from build123d import *

# Parameters (mm, degrees)
EXTRUDE_1_DEPTH     = 40
CUT_EXTRUDE_1_REACH = 130.577
CUT_EXTRUDE_2_REACH = 130.577


with BuildPart() as part:
    # 草图1 → 凸台-拉伸1 (new body)
    with BuildSketch(Plane(origin=(0, 0, 0), x_dir=(0, 0, -1), z_dir=(1, 0, 0))):
        Polygon((0, 0), (0, 114), (44, 114), (44, 110), (4, 110), (4, 0), align=None)
    extrude(amount=EXTRUDE_1_DEPTH)

    # 草图2 → 切除-拉伸1 (cut, up to next)
    with BuildSketch(Plane(origin=(0, 114, 0), x_dir=(1, 0, 0), z_dir=(0, 1, 0)), mode=Mode.PRIVATE) as cut_extrude_1_sk1:
        with BuildLine():
            Line((17, 32), (17, 17))
            ThreePointArc((17, 17), (20, 14), (23, 17))
            Line((23, 17), (23, 32))
            ThreePointArc((23, 32), (20, 35), (17, 32))
        make_face()
    cut_extrude_1_tool1 = extrude(cut_extrude_1_sk1.sketch, amount=-CUT_EXTRUDE_1_REACH, mode=Mode.PRIVATE) & part.part
    add(cut_extrude_1_tool1.solids().sort_by_distance((20, 114, -24.5))[0], mode=Mode.SUBTRACT)

    # 草图3 → 切除-拉伸2 (cut, up to next)
    with BuildSketch(Plane.XY, mode=Mode.PRIVATE) as cut_extrude_2_sk1:
        with BuildLine():
            Line((23.5, 15), (23.5, 35))
            ThreePointArc((23.5, 35), (20, 38.5), (16.5, 35))
            Line((16.5, 35), (16.5, 15))
            ThreePointArc((16.5, 15), (20, 11.5), (23.5, 15))
        make_face()
    cut_extrude_2_tool1 = extrude(cut_extrude_2_sk1.sketch, amount=-CUT_EXTRUDE_2_REACH, mode=Mode.PRIVATE) & part.part
    add(cut_extrude_2_tool1.solids().sort_by_distance((20, 25, 0))[0], mode=Mode.SUBTRACT)


solid = part.part
Here's how the part is built. I have some questions about the finished solid (model axes, mm). A direction names the side the tool comes from. Coordinates: 2 decimals unless noted, no trailing zeros. Write each loop counter-clockwise with the first axis right and the second up, starting at its lowest first coordinate (ties: lowest second). Pieces come first, ordered by that corner, then holes. Notation, with made-up numbers: (47.5, -40) - (58.5, -40) arc R18 ccw to (58.5, -11) - close; hole circle Ø5 at (76, 17). An arc over 180 degrees is marked (long way). Use one line per item in the form item = value.
1) Suppose I cut it at D-D, the plane y = 47. Write out the boundary of the cut face in (x, z), plus the area to 3 significant figures.
Solved:
outline = (0, -4) - (40, -4) - (40, 0) - (0, 0) - close
area = 160 mm2
2) I need wall thicknesses on line 1 (Y direction, x = 22, z = -41); line 2 (Z direction, x = 31, y = 83). Which ranges of each line are inside material? Lowest first, please.
Solved:
line_1 = 110 to 114
line_2 = -4 to 0
3) Suppose I cut it at B-B, the plane y = 19. Write out the boundary of the cut face in (x, z).
Solved:
outline = (0, -4) - (16.5, -4) - (16.5, 0) - (0, 0) - close; (23.5, -4) - (40, -4) - (40, 0) - (23.5, 0) - close
4) I'm going to push flat-ended pins straight in: P1, Ø4, axis at x = 11, z = -30.5, coming from the -Y side; P2, Ø12, axis at x = 24, y = 46.5, coming from the -Z side. Where does each tip first touch, or does it pass through?
Solved:
P1 = 110
P2 = -4
5) Suppose I cut it at C-C, the plane x = 20. Write out the boundary of the cut face in (y, z).
Solved:
outline = (0, -4) - (11.5, -4) - (11.5, 0) - (0, 0) - close; (38.5, -4) - (110, -4) - (110, -14) - (114, -14) - (114, 0) - (38.5, 0) - close; (110, -44) - (114, -44) - (114, -35) - (110, -35) - close
6) Suppose I cut it at A-A, the plane z = -27. Write out the boundary of the cut face in (x, y).
Solved:
outline = (0, 110) - (17, 110) - (17, 114) - (0, 114) - close; (23, 110) - (40, 110) - (40, 114) - (23, 114) - close
7) Thinking about a two-plate mould opening in X: for faces 1 (the flat face through (20, 56, 0)), 2 (the flat face through (40, 74, -3)), 3 (the flat face through (23, 112, -24)), which applies, released by +X, released by -X, zero draft, split by the parting line, or undercut?
Solved:
face_1 = zero draft
face_2 = released by +X
face_3 = undercut
8) On a 3-axis mill with a long thin cutter (end or side, diameter ignored), from which of +Z, -Z, +X, -X, +Y, -Y can I reach the whole of each face in a straight line? I mean faces 4 (the flat face through (17, 112, -25)), 5 (the cylindrical face through (19.9, 11.5, -2)), 6 (the flat face through (20, 56, -4)). Say none if no direction works.
Solved:
face_4 = +Y, -Y
face_5 = +Z, -Z
face_6 = -Z, +X, -X, -Y
